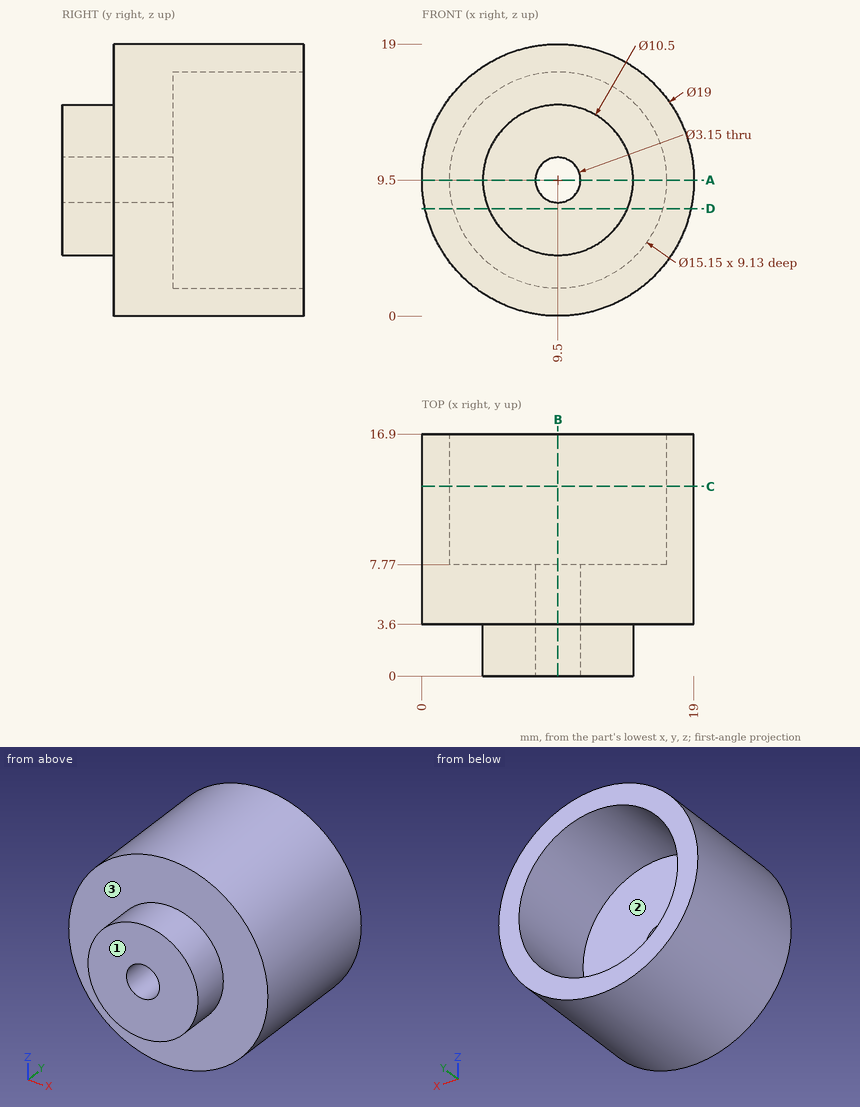
Verification items for this drawing (mm, ordinates from the low corner). A direction names the side the tool comes from. Coordinates: 2 decimals unless noted, no trailing zeros. Write each loop counter-clockwise with the first axis right and the second up, starting at its lowest first coordinate (ties: lowest second). Pieces come first, ordered by that corner, then holes. Notation, with made-up numbers: M -29,-19.75 L -13,-19.75 A7 cw -13,-15.75 Z; hole C 37,30.25 d4. An arc over 180 degrees is marked long. Use one line per item in the form item = value. Start each with the question number.
1) Set-up check for the marked faces 1, 2 and 3: record each of +Z, -Z, +X, -X, +Y, -Y from which the full face is reachable in a straight line by a thin tool's end or side.
2) Thickness scan on probe 1 along Z at (x, y) = (9.5, 3.25) (3 decimals); probe 2 along X at (y, z) = (12.75, 9.5) (3 decimals); probe 3 along Z at (x, y) = (9.5, 5.5) (3 decimals). Record the ranges inside material, lowest first. Write a range as from..to.
3) Go/stop test with flat-tipped pins: pin 1 Ø3 at (x, y) = (4, 6) entering from +Z; pin 2 Ø4 at (x, z) = (8.5, 3.5) entering from +Y; pin 3 Ø2 at (x, z) = (3, 4.5) entering from -Y; pin 4 Ø3 at (x, y) = (5, 10) entering from +Z. Record where each tip stops, or that it passes through.
4) Section check C-C on y = 13.25. Enter the section's corners in (x, z) (3 decimals).
5) Section check D-D on z = 7.5. Enter the section's corners in (x, y).
6) Section check A-A on z = 9.5. Enter the section's corners in (x, y) (3 decimals), and give its area (3 significant figures).
7) Section check B-B on x = 9.5. Enter the section's corners in (y, z) (3 decimals).
Responses:
q1.face_1 = +Z, -Z, +X, -X, -Y
q1.face_2 = +Y
q1.face_3 = -Y
q2.probe_1 = 4.25..7.925, 11.075..14.75
q2.probe_2 = 0..1.925, 17.075..19
q2.probe_3 = 0..7.925, 11.075..19
q3.pin_1 = 18.12
q3.pin_2 = 16.9
q3.pin_3 = 3.6
q3.pin_4 = 18.51
q4.outline = C 9.5,9.5 d19; hole C 9.5,9.5 d15.15
q5.outline = M 0.21,3.6 L 4.65,3.6 L 4.65,0 L 14.35,0 L 14.35,3.6 L 18.79,3.6 L 18.79,16.9 L 16.81,16.9 L 16.81,7.77 L 2.19,7.77 L 2.19,16.9 L 0.21,16.9 Z
q6.outline = M 0,3.6 L 4.25,3.6 L 4.25,0 L 7.925,0 L 7.925,7.77 L 1.925,7.77 L 1.925,16.9 L 0,16.9 Z; M 11.075,0 L 14.75,0 L 14.75,3.6 L 19,3.6 L 19,16.9 L 17.075,16.9 L 17.075,7.77 L 11.075,7.77 Z
q6.area = 128 mm2
q7.outline = M 0,4.25 L 3.6,4.25 L 3.6,0 L 16.9,0 L 16.9,1.925 L 7.77,1.925 L 7.77,7.925 L 0,7.925 Z; M 0,11.075 L 7.77,11.075 L 7.77,17.075 L 16.9,17.075 L 16.9,19 L 3.6,19 L 3.6,14.75 L 0,14.75 Z
